For this review, take the finished solid that the model builds, in its own axes (mm). Face numbers are marked on the shaded views. A direction names the side the tool comes from. Give positions to 0.01 mm unless a question says otherwise; leave off trailing zeros. Loops run counter-clockwise (first coordinate to the right, second up) from the corner with the lowest first, then second, coordinate; pieces in that order, holes last. Notation, with made-up numbers: (55.5, 22) - (91.5, 22) arc R25 cw to (91.5, 37) - close; hole circle Ø2 at (19, 84). An arc over 180 degrees is marked (long way). Answer in a Markdown table with one row per item.
```python
from build123d import *

# Parameters (mm, degrees)
EXTRUDE_1_DEPTH     = 78
EXTRUDE_2_DEPTH     = 78
EXTRUDE_4_DEPTH     = 6
CUT_EXTRUDE_3_DEPTH = 80
CUT_EXTRUDE_4_DEPTH = 160.514889587
CUT_EXTRUDE_5_DEPTH = 170.32217811
SKETCH_10_W         = 24
SKETCH_10_H         = 10
CUT_EXTRUDE_6_DEPTH = 1.5
FILLET_1_R          = 4
FILLET_START        = -45
FILLET_6_DEPTH      = 77
FILLET_START_2      = -39
FILLET_6_2_DEPTH    = 78


with BuildPart() as part:
    # 草图1 → 凸台-拉伸1 (new body)
    with BuildSketch(Plane(origin=(-39, 0, 0), x_dir=(0, 0, -1), z_dir=(1, 0, 0))):
        Polygon((55, 0), (-55, 0), (-55, 8), (45, 8), (45, 20), (55, 20), align=None)
    extrude(amount=EXTRUDE_1_DEPTH)

    # 草图2 → 凸台-拉伸2 (add)
    with BuildSketch(Plane(origin=(-39, 0, 0), x_dir=(0, 0, -1), z_dir=(1, 0, 0))):
        Polygon((-17.5, 0), (-49.042, 118), (-54.81, 116.346), (-21.45, 0), align=None)
    extrude(amount=EXTRUDE_2_DEPTH)

    # 草图4 → 凸台-拉伸4 (add)
    with BuildSketch(Plane(origin=(33, 0, 0), x_dir=(0, 0, -1), z_dir=(1, 0, 0))):
        Polygon((-20, 6), (-40, 6), (-32, 45), align=None)
    extrude_4 = extrude(amount=EXTRUDE_4_DEPTH)

    # 镜向1: 凸台-拉伸4 across plane
    add(extrude_4.mirror(Plane(origin=(0, 0, 0), x_dir=(0, 0, 1), z_dir=(1, 0, 0))))

    # 草图7 → 切除-拉伸3 (cut)
    with BuildSketch(Plane(origin=(-40, 0, 0), x_dir=(0, 0, -1), z_dir=(1, 0, 0))):
        with BuildLine():
            Line((-16, 6), (-16, 28))
            ThreePointArc((-16, 28), (-24, 36), (-32, 28))
            Line((-32, 28), (-32, 6))
            Line((-32, 6), (-16, 6))
        make_face()
    extrude(amount=CUT_EXTRUDE_3_DEPTH, mode=Mode.SUBTRACT)

    # 草图8 → 切除-拉伸4 (cut, through all)
    with BuildSketch(Plane.XY.offset(45)):
        with BuildLine():
            Line((-15, 58), (15, 58))
            ThreePointArc((15, 58), (17.121320344, 58.878679656), (18, 61))
            Line((18, 61), (18, 63))
            ThreePointArc((18, 63), (17.121320344, 65.121320344), (15, 66))
            Line((15, 66), (-15, 66))
            ThreePointArc((-15, 66), (-17.121320344, 65.121320344), (-18, 63))
            Line((-18, 63), (-18, 61))
            ThreePointArc((-18, 61), (-17.121320344, 58.878679656), (-15, 58))
        make_face()
        with BuildLine():
            Line((-15, 76), (15, 76))
            ThreePointArc((15, 76), (17.121320344, 76.878679656), (18, 79))
            Line((18, 79), (18, 81))
            ThreePointArc((18, 81), (17.121320344, 83.121320344), (15, 84))
            Line((15, 84), (-15, 84))
            ThreePointArc((-15, 84), (-17.121320344, 83.121320344), (-18, 81))
            Line((-18, 81), (-18, 79))
            ThreePointArc((-18, 79), (-17.121320344, 76.878679656), (-15, 76))
        make_face()
        with BuildLine():
            Line((-15, 94), (15, 94))
            ThreePointArc((15, 94), (17.121320344, 94.878679656), (18, 97))
            Line((18, 97), (18, 99))
            ThreePointArc((18, 99), (17.121320344, 101.121320344), (15, 102))
            Line((15, 102), (-15, 102))
            ThreePointArc((-15, 102), (-17.121320344, 101.121320344), (-18, 99))
            Line((-18, 99), (-18, 97))
            ThreePointArc((-18, 97), (-17.121320344, 94.878679656), (-15, 94))
        make_face()
    extrude(amount=-CUT_EXTRUDE_4_DEPTH, mode=Mode.SUBTRACT)

    # 草图9 → 切除-拉伸5 (cut, through all)
    with BuildSketch(Plane.XY.offset(60)):
        with BuildLine():
            Line((-15, 58), (15, 58))
            ThreePointArc((15, 58), (17.121320344, 58.878679656), (18, 61))
            Line((18, 61), (18, 63))
            ThreePointArc((18, 63), (17.121320344, 65.121320344), (15, 66))
            Line((15, 66), (-15, 66))
            ThreePointArc((-15, 66), (-17.121320344, 65.121320344), (-18, 63))
            Line((-18, 63), (-18, 61))
            ThreePointArc((-18, 61), (-17.121320344, 58.878679656), (-15, 58))
        make_face()
        with BuildLine():
            Line((-15, 76), (15, 76))
            ThreePointArc((15, 76), (17.121320344, 76.878679656), (18, 79))
            Line((18, 79), (18, 81))
            ThreePointArc((18, 81), (17.121320344, 83.121320344), (15, 84))
            Line((15, 84), (-15, 84))
            ThreePointArc((-15, 84), (-17.121320344, 83.121320344), (-18, 81))
            Line((-18, 81), (-18, 79))
            ThreePointArc((-18, 79), (-17.121320344, 76.878679656), (-15, 76))
        make_face()
        with BuildLine():
            Line((-15, 94), (15, 94))
            ThreePointArc((15, 94), (17.121320344, 94.878679656), (18, 97))
            Line((18, 97), (18, 99))
            ThreePointArc((18, 99), (17.121320344, 101.121320344), (15, 102))
            Line((15, 102), (-15, 102))
            ThreePointArc((-15, 102), (-17.121320344, 101.121320344), (-18, 99))
            Line((-18, 99), (-18, 97))
            ThreePointArc((-18, 97), (-17.121320344, 94.878679656), (-15, 94))
        make_face()
    extrude(amount=-CUT_EXTRUDE_5_DEPTH, mode=Mode.SUBTRACT)

    # 草图10 → 切除-拉伸6 (cut)
    with BuildSketch(Plane(origin=(0, 0, 0), x_dir=(1, 0, 0), z_dir=(0, 1, 0))):
        with Locations((0, 45)):
            Rectangle(SKETCH_10_W, SKETCH_10_H)
        with Locations((0, -45)):
            Rectangle(SKETCH_10_W, SKETCH_10_H)
    extrude(amount=CUT_EXTRUDE_6_DEPTH, mode=Mode.SUBTRACT)

    # 圆角1
    fillet_1_edges = [part.edges().sort_by_distance(p)[0] for p in [
        (0, 20, -45),
        (0, 20, -55),
        (39, 4, 55),
        (39, 10, -55),
        (-39, 4, 55),
        (-39, 10, -55),
    ]]
    fillet(fillet_1_edges, radius=FILLET_1_R)

    # 圆角6: read off the stored shape, not the designer's step
    # 圆角6 outline → 圆角6 (cut)
    with BuildSketch(Plane.XY.offset(FILLET_START)):
        with BuildLine():
            Line((-39, 8), (-39, 4))
            ThreePointArc((-39, 4), (-37.828427125, 6.828427125), (-35, 8))
            Line((-35, 8), (-39, 8))
        make_face()
        with BuildLine():
            Line((39, 8), (35, 8))
            ThreePointArc((35, 8), (37.828427125, 6.828427125), (39, 4))
            Line((39, 4), (39, 8))
        make_face()
    extrude(amount=FILLET_6_DEPTH, mode=Mode.SUBTRACT)

    # Fillet 6 2 outline → Fillet 6 2 (cut)
    with BuildSketch(Plane.YZ.offset(FILLET_START_2)):
        with BuildLine():
            Line((8, 55), (4, 55))
            ThreePointArc((4, 55), (6.828427125, 53.828427125), (8, 51))
            Line((8, 51), (8, 55))
        make_face()
    extrude(amount=FILLET_6_2_DEPTH, mode=Mode.SUBTRACT)


solid = part.part
```
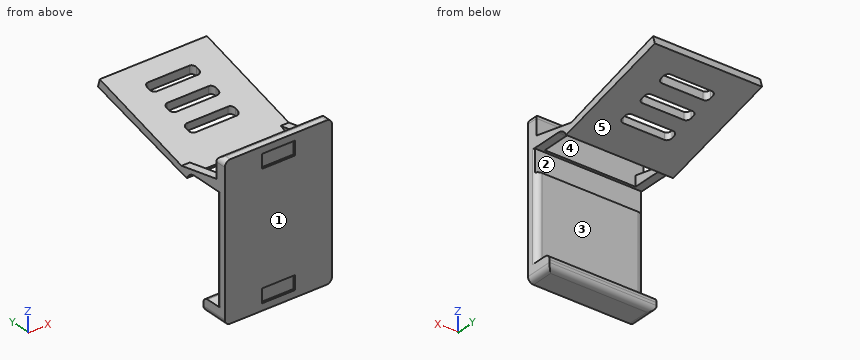
1. We need section C-C, the plane z = 11. Give the boundary of the cut face in (x, y).
Values:
| item | result |
|---|---|
| outline | (-39, 0) - (39, 0) - (39, 4) arc R4 ccw to (35, 8) - (-35, 8) arc R4 ccw to (-39, 4) - close |
2. For the marked faces 4 and 5, list the 3-axis set-ups (+Z, -Z, +X, -X, +Y, -Y) from which the entire face can be reached by the end or side of a thin tool; tool diameter is ignored.
Values:
| item | result |
|---|---|
| face 4 | +Z |
| face 5 | -Z, +X, -X, +Y |
3. We need section A-A, the plane x = -23. Give the boundary of the cut face in (y, z).
Values:
| item | result |
|---|---|
| outline | (0, -55) - (16, -55) arc R4 ccw to (20, -51) - (20, -49) arc R4 ccw to (16, -45) - (8, -45) - (8, 16) - (6, 16) - (6, 32) - (8, 32) - (8, 51) arc R4 ccw to (4, 55) - (0, 55) - close; (32.34, 30.72) arc R8 cw to (35.43, 26.97) - (118, 49.04) - (116.35, 54.81) - close |
4. Wall thickness on line 1 (Y direction, x = 18.5, z = -22); line 2 (Y direction, x = 9, z = 19); line 3 (Z direction, x = 27, y = 13): over which ranges is each line inside the solid? List them lowest first. Write a range as [from, to].
Values:
| item | result |
|---|---|
| line 1 | y = [0, 8] |
| line 2 | y = [0, 6] |
| line 3 | z = [-55, -45] |
5. Clearance check with flat-ended pins moving along their axes: pin 1 (5 mm diameter, centred on x = 13, y = 30.5, fed in from -Z) (3 decimals); pin 2 (8 mm diameter, centred on x = 7.5, z = 22, fed in from +Y); pin 3 (2 mm diameter, centred on x = -14.5, y = 94.5, fed in from +Z). State where each tip first meets the part, or that it passes through.
Values:
| item | result |
|---|---|
| pin 1 | stops at z = 30.245 |
| pin 2 | stops at y = 6 |
| pin 3 | stops at z = 48.41 |
6. Mouldability with a two-part tool opening along Y and no side actions: class the marked faces 1, 2 and 3 as released by +Y, released by -Y, zero draft, split by the parting line, or undercut.
Values:
| item | result |
|---|---|
| face 1 | released by -Y |
| face 2 | undercut |
| face 3 | released by +Y |
7. We need section D-D, the plane y = 50.5. Give the boundary of the cut face in (x, z), and give its area (3 significant figures).
Values:
| item | result |
|---|---|
| outline | (-39, 31) - (39, 31) - (39, 35.93) - (-39, 35.93) - close |
| area | 385 mm^2 |
8. We need section B-B, the plane x = -3.5. Count the separate pieces of the cut face and the enclosed holes in it, and give its area (3 significant figures).
Values:
| item | result |
|---|---|
| separate pieces | 5 |
| enclosed holes | 0 |
| area | 1,250 mm^2 |
